Work out the finished part from the listing and answer in its coordinate system (mm). Face numbers are marked on the shaded views. Give positions to 0.01 mm unless a question says otherwise; leave off trailing zeros. Order: outer loops, then holes, each group sorted by start corner. A loop starts at its lowest first (then second) coordinate and runs counter-clockwise, first axis right, second up.
```python
from build123d import *

# Parameters (mm, degrees)
F0_R     = 31.75
F0_R_2   = 13.0175
F1_DEPTH = 38.1
F2_SIZE  = 2.54
F3_SIZE  = 0.762


with BuildPart() as f1:
    # F0 (on Top) → F1 (new body)
    with BuildSketch(Plane.XY):
        Circle(F0_R)
        Circle(F0_R_2, mode=Mode.SUBTRACT)
    extrude(amount=F1_DEPTH)

    # F2
    f2_edges = [f1.edges().sort_by_distance(p)[0] for p in [
        (-31.75, 0, 38.1),
    ]]
    chamfer(f2_edges, length=F2_SIZE)

    # F3
    f3_edges = [f1.edges().sort_by_distance(p)[0] for p in [
        (-13.0175, 0, 38.1),
        (-13.0175, 0, 0),
    ]]
    chamfer(f3_edges, length=F3_SIZE)


solid = f1.part
```
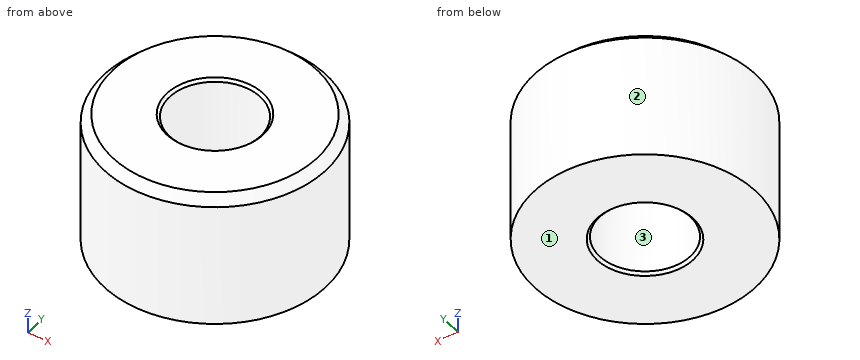
1. Straight lines are drawn through the part: probe 1 along Y at (x, z) = (0, 15); probe 2 along Y at (x, z) = (-3.5, 9); probe 3 along X at (y, z) = (-9.5, 33.5). For each, find the intervals that lie inside material, in ascending order.
Findings below:
probe 1: y = -31.75 to -13.02, 13.02 to 31.75
probe 2: y = -31.56 to -12.54, 12.54 to 31.56
probe 3: x = -30.3 to -8.9, 8.9 to 30.3
2. Given P1, Ø5, axis at y = -4.5, z = 21, coming from the +X side; P2, Ø15.5, axis at x = 0, y = 0, coming from the -Z side; P3, Ø1.5, axis at x = 9.5, z = 4.5, coming from the -Y side; P4, Ø10, axis at x = -17, z = 34, coming from the +Y side, each flat-ended and moving along its own axis, determine where each tip first touches the part or whether it passes through.
Findings below:
P1: stops at x = 31.69
P2: passes through
P3: stops at y = -30.52
P4: stops at y = 29.39
3. The part is cut by section A-A (x = 0). Write down the section's boundary in (y, z).
Findings below:
outline: (-31.75, 0) - (-13.78, 0) - (-13.02, 0.76) - (-13.02, 37.34) - (-13.78, 38.1) - (-29.21, 38.1) - (-31.75, 35.56) - close; (13.02, 0.76) - (13.78, 0) - (31.75, 0) - (31.75, 35.56) - (29.21, 38.1) - (13.78, 38.1) - (13.02, 37.34) - close
4. The mould has two halves that part along Y. Classify the marked faces 1, 2 and 3: pulls with the +Y half, pulls with the -Y half, needs draft (parallel to the pull), parting line crosses it, or undercut.
Findings below:
face 1: needs draft
face 2: parting line crosses it
face 3: undercut
